from build123d import *

# Parameters (mm, degrees)
SKETCH1_R           = 1.8288
BOSS_EXTRUDE1_DEPTH = 9.525
SKETCH2_R           = 3.4925
BOSS_EXTRUDE2_DEPTH = 1.27
DOME1_FACE_RADIUS   = 3.4925
DOME1_HEIGHT        = 1.27
SKETCH3_W           = 2.4384
SKETCH3_H           = 2.4384
CUT_EXTRUDE1_DEPTH  = 2.032


with BuildPart() as part:
    # Sketch1 → Boss-Extrude1 (new body)
    with BuildSketch(Plane(origin=(0, 0, 0), x_dir=(1, 0, 0), z_dir=(0, 1, 0))):
        with Locations(Location((0, 0, 0), (0, 0, 270))):
            Circle(SKETCH1_R)
    extrude(amount=-BOSS_EXTRUDE1_DEPTH)

    # Sketch2 → Boss-Extrude2 (add)
    with BuildSketch(Plane(origin=(0, 0, 0), x_dir=(1, 0, 0), z_dir=(0, 1, 0))):
        with Locations(Location((0, 0, 0), (0, 0, 270))):
            Circle(SKETCH2_R)
    extrude(amount=BOSS_EXTRUDE2_DEPTH)

    # Dome1: a dome of height H over a round flat face of radius A is a cap of a sphere of radius (A * A + H * H) / (2 * H)
    dome1_r = (DOME1_FACE_RADIUS * DOME1_FACE_RADIUS + DOME1_HEIGHT * DOME1_HEIGHT) / (2 * DOME1_HEIGHT)
    dome1_base = Plane((0, 1.27, 0), z_dir=(0, 1, 0))
    with Locations(dome1_base.offset(DOME1_HEIGHT - dome1_r)):
        dome1_ball = Sphere(dome1_r, mode=Mode.PRIVATE)
    add(split(dome1_ball, bisect_by=dome1_base, keep=Keep.TOP, mode=Mode.PRIVATE))

    # Sketch3 → Cut-Extrude1 (cut)
    with BuildSketch(Plane(origin=(0, 2.54, 0), x_dir=(1, 0, 0), z_dir=(0, 1, 0))):
        Rectangle(SKETCH3_W, SKETCH3_H)
    extrude(amount=-CUT_EXTRUDE1_DEPTH, mode=Mode.SUBTRACT)


solid = part.part
Source: CAD feature listing. Evaluate the final solid. Frame: model axes, mm. A direction names the side the tool comes from. Coordinates: 2 decimals unless noted, no trailing zeros. Write each loop counter-clockwise with the first axis right and the second up, starting at its lowest first coordinate (ties: lowest second). Pieces come first, ordered by that corner, then holes. Notation, with made-up numbers: M 51.25,16 L 96.25,16 A17 cw 96.25,29 Z; hole C -34.5,-6.5 d11. An arc over 180 degrees is marked long. Use a Markdown table: item, result.
1) Section C-C, the plane y = -1.75. Output: boundary loops of the cut face in (x, z), then the cut area to 3 significant figures.
Conclusion:
| item | result |
|---|---|
| outline | C 0,0 d3.66 |
| area | 10.5 mm^2 |
2) Section B-B, the plane x = 0.5. Output: boundary loops of the cut face in (y, z) (3 decimals).
Conclusion:
| item | result |
|---|---|
| outline | M -9.525,-1.759 L 0,-1.759 L 0,-3.457 L 1.27,-3.457 A5.414 ccw 2.378,-1.219 L 0.508,-1.219 L 0.508,1.219 L 2.378,1.219 A5.414 ccw 1.27,3.457 L 0,3.457 L 0,1.759 L -9.525,1.759 Z |
3) Mould query, pull axis X, two halves, no side actions, for faces 1 (the flat face through (-2, 0, 2)), 2 (the flat face through (1.219, 1, 0)), 3 (the cylindrical face through (-1.113, -4.696, -1.451)). Classes: pulls with the +X half, pulls with the -X half, needs draft (parallel to the pull), parting line crosses it, or undercut.
Conclusion:
| item | result |
|---|---|
| face 1 | needs draft |
| face 2 | undercut |
| face 3 | parting line crosses it |
4) Section D-D, the plane x = 1.5. Output: boundary loops of the cut face in (y, z) (3 decimals), then the cut area to 3 significant figures.
Conclusion:
| item | result |
|---|---|
| outline | M -9.525,-1.046 L 0,-1.046 L 0,-3.154 L 1.27,-3.154 A5.226 ccw 1.27,3.154 L 0,3.154 L 0,1.046 L -9.525,1.046 Z |
| area | 32.5 mm^2 |
5) Reachability of faces 4 (the flat face through (-1.219, 1, 0)), 5 (the cylindrical face through (3.463, 0.626, -0.455)) from +Z, -Z, +X, -X, +Y, -Y: full face, straight path, thin tool, end or side. Return the list, or none.
Conclusion:
| item | result |
|---|---|
| face 4 | +Y |
| face 5 | +Y, -Y |
6) Ray query, L1, parallel to Y at x = 0.25, z = 0.5 (3 decimals); L2, parallel to X at y = -6.25, z = 0; L3, parallel to Y at x = 3, z = -1. Return the intervals inside material, ascending.
Conclusion:
| item | result |
|---|---|
| L1 | y = -9.525 to 0.508 |
| L2 | x = -1.83 to 1.83 |
| L3 | y = 0 to 1.53 |
7) First-contact query: pin 1 Ø1.5 at (x, z) = (-1.5, -1.5) entering from +Y. Flat tip, straight axial feed; report the tip coordinate or a pass-through.
Conclusion:
| item | result |
|---|---|
| pin 1 | stops at y = 2.34 |
8) Section A-A, the plane z = 0. Output: boundary loops of the cut face in (x, y) (1 decimal).
Conclusion:
| item | result |
|---|---|
| outline | M -3.5,0 L -1.8,0 L -1.8,-9.5 L 1.8,-9.5 L 1.8,0 L 3.5,0 L 3.5,1.3 A5.4 ccw 1.2,2.4 L 1.2,0.5 L -1.2,0.5 L -1.2,2.4 A5.4 ccw -3.5,1.3 Z |
